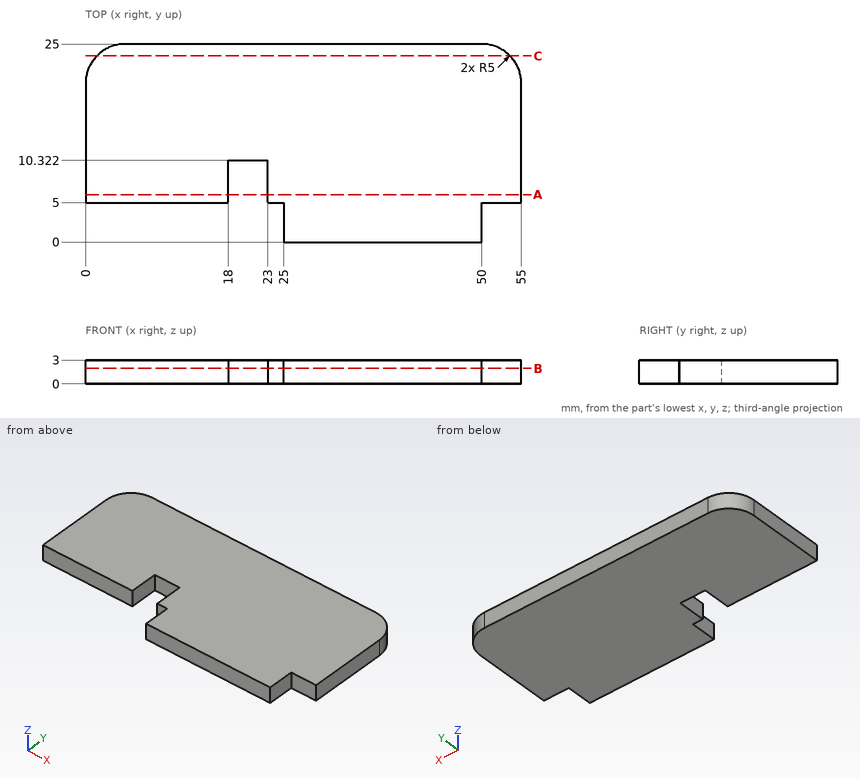
Here's the drawing with two shaded views (mm, measured from the low corner). I have some questions. Give positions to 0.01 mm unless a question says otherwise; leave off trailing zeros. Loops run counter-clockwise (first coordinate to the right, second up) from the corner with the lowest first, then second, coordinate; pieces in that order, holes last. Notation, with made-up numbers: M 17.25,69.5 L 51.25,69.5 A19 ccw 51.25,98.5 Z; hole C 62.25,-40 d1. An arc over 180 degrees is marked long. One line per item, written item: value.
1) Imagine slicing it at A-A on y = 6. Write out the boundary of the cut face in (x, z), and give its area (3 significant figures).
Geometry check:
outline: M 0,0 L 18,0 L 18,3 L 0,3 Z; M 23,0 L 55,0 L 55,3 L 23,3 Z
area: 150 mm²
2) Imagine slicing it at C-C on y = 23.5. Write out the boundary of the cut face in (x, z).
Geometry check:
outline: M 1.43,0 L 53.57,0 L 53.57,3 L 1.43,3 Z
3) Please list where these lines run through material, in increasing order: line 1 (X direction, y = 8.5, z = 2.05); line 2 (Y direction, x = 18.5, z = 1.9); line 3 (X direction, y = 1.75, z = 2.4).
Geometry check:
line 1: x = 0 to 18, 23 to 55
line 2: y = 10.32 to 25
line 3: x = 25 to 50
4) Imagine slicing it at B-B on z = 1.95. Write out the boundary of the cut face in (x, y).
Geometry check:
outline: M 0,5 L 18,5 L 18,10.32 L 23,10.32 L 23,5 L 25,5 L 25,0 L 50,0 L 50,5 L 55,5 L 55,20 A5 ccw 50,25 L 5,25 A5 ccw 0,20 Z
5) I'm going to push flat-ended pins straight in: pin 1 (1.5 mm diameter, centred on y = 3, z = 1, fed in from +X); pin 2 (0.9 mm diameter, centred on y = 2.5, z = 1.5, fed in from -X). Where does each tip first touch, or does it pass through?
Geometry check:
pin 1: stops at x = 50
pin 2: stops at x = 25
